```python
from build123d import *

# Parameters (mm, degrees)
F4_W     = 203.2
F4_H     = 101.6
F5_DEPTH = 127
F1_DEPTH = 76.2
F3_DEPTH = 76.2


with BuildPart() as f5:
    # F4 (on Top) → F5 (new body)
    with BuildSketch(Plane.XY):
        with Locations((45.487865, 3.072385)):
            Rectangle(F4_W, F4_H)
    extrude(amount=F5_DEPTH)

    # F0 (on face) → F1 (cut)
    with BuildSketch(Plane.YZ.offset(147.087865)):
        Polygon((-47.727615, 50.8), (28.472385, 127), (-47.727615, 127), align=None)
    extrude(amount=-F1_DEPTH, mode=Mode.SUBTRACT)

    # F2 (on face) → F3 (cut)
    with BuildSketch(Plane(origin=(-56.112135, 0, 0), x_dir=(0, -1, 0), z_dir=(-1, 0, 0))):
        Polygon((-27.847318, 127), (47.727615, 50.8), (47.727615, 127), align=None)
    extrude(amount=-F3_DEPTH, mode=Mode.SUBTRACT)


solid = f5.part
```
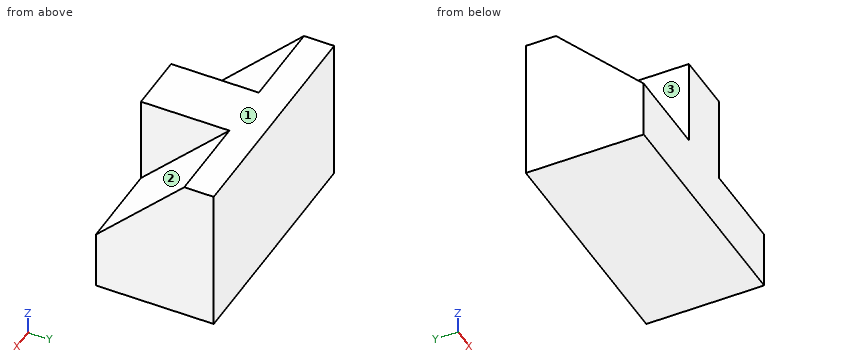
Here's how the part is built. I have some questions about the finished solid (model axes, mm). Face numbers are marked on the shaded views. A direction names the side the tool comes from. Give positions to 0.01 mm unless a question says otherwise; leave off trailing zeros. Write each loop counter-clockwise with the first axis right and the second up, starting at its lowest first coordinate (ties: lowest second). Pieces come first, ordered by that corner, then holes.
(1) If I drill on L1, parallel to X at y = -41, z = 71; L2, parallel to Z at x = 123, y = -26; L3, parallel to Z at x = -29, y = 23, over which ranges is the centre line in solid material (lowest first)?
Output values:
L1: x = 20.09 to 70.89
L2: z = 0 to 72.53
L3: z = 0 to 122.11
(2) Imagine slicing it at B-B, the plane y = -39. Write out the boundary of the cut face in (x, z).
Output values:
outline: (-56.11, 0) - (147.09, 0) - (147.09, 59.53) - (70.89, 59.53) - (70.89, 127) - (20.09, 127) - (20.09, 59.6) - (-56.11, 59.6) - close
(3) Imagine slicing it at A-A, the plane x = 80.5. Write out the boundary of the cut face in (y, z).
Output values:
outline: (-47.73, 0) - (53.87, 0) - (53.87, 127) - (28.47, 127) - (-47.73, 50.8) - close
(4) On a 3-axis mill with a long thin cutter (end or side, diameter ignored), from which of +Z, -Z, +X, -X, +Y, -Y can I reach the whole of each face in a straight line? I mean the marked faces 1, 2 and 3. Say none if no direction works.
Output values:
face 1: +Z, +X, -X, +Y, -Y
face 2: +Z, +X, -Y
face 3: +Z, -X, -Y
(5) Will this pin go through, and if not, where does the flat tip stop? pin 1 (1 mm diameter, centred on x = 3.5, y = -12.5, fed in from +Z).
Output values:
pin 1: stops at z = 86.82
(6) Imagine slicing it at C-C, the plane z = 65.5. Write out the boundary of the cut face in (x, y).
Output values:
outline: (-56.11, -33.15) - (20.09, -33.15) - (20.09, -47.73) - (70.89, -47.73) - (70.89, -33.03) - (147.09, -33.03) - (147.09, 53.87) - (-56.11, 53.87) - close
